Build history of the part. All positions in model axes, mm. A direction names the side the tool comes from. Round coordinates to 2 decimals unless told otherwise and drop trailing zeros. Write each loop counter-clockwise with the first axis right and the second up, starting at its lowest first coordinate (ties: lowest second). Pieces come first, ordered by that corner, then holes.
from build123d import *

# Parameters (mm, degrees)
F0_R     = 3
F1_DEPTH = 7.5
F0_R_2   = 2.35
F2_DEPTH = 7
F3_DEPTH = 0.5
F4_DEPTH = 7
F5_DEPTH = 0.5


with BuildPart() as f1:
    # F0 (on Top) → F1 (new body)
    with BuildSketch(Plane.XY):
        with BuildLine():
            ThreePointArc((-61.751105, -13.001984), (-60.682045, -15.582924), (-58.101105, -16.651984))
            Line((-58.101105, -16.651984), (5.748895, -16.651984))
            ThreePointArc((5.748895, -16.651984), (8.329835, -15.582924), (9.398895, -13.001984))
            ThreePointArc((9.398895, -13.001984), (8.329835, -10.421045), (5.748895, -9.351984))
            Line((5.748895, -9.351984), (-58.101105, -9.351984))
            ThreePointArc((-58.101105, -9.351984), (-60.682045, -10.421045), (-61.751105, -13.001984))
        make_face()
        with Locations((-58.101105, -13.001984)):
            Circle(F0_R, mode=Mode.SUBTRACT)
        with Locations((-50.101105, -13.001984)):
            Circle(F0_R, mode=Mode.SUBTRACT)
        with Locations((-42.101105, -13.001984)):
            Circle(F0_R, mode=Mode.SUBTRACT)
        with Locations((-34.101105, -13.001984)):
            Circle(F0_R, mode=Mode.SUBTRACT)
        with Locations((-26.101105, -13.001984)):
            Circle(F0_R, mode=Mode.SUBTRACT)
        with Locations((-18.101105, -13.001984)):
            Circle(F0_R, mode=Mode.SUBTRACT)
        with Locations((-10.101105, -13.001984)):
            Circle(F0_R, mode=Mode.SUBTRACT)
        with Locations((-2.101105, -13.001984)):
            Circle(F0_R, mode=Mode.SUBTRACT)
        with Locations((5.898895, -13.001984)):
            Circle(F0_R, mode=Mode.SUBTRACT)
    extrude(amount=F1_DEPTH)

    # F0 (on Top) → F2 (join)
    with BuildSketch(Plane.XY):
        with Locations((5.898895, -13.001984)):
            Circle(F0_R)
        with Locations((5.898895, -13.001984)):
            Circle(F0_R_2, mode=Mode.SUBTRACT)
    extrude(amount=F2_DEPTH)

    # F0 (on Top) → F3 (cut)
    with BuildSketch(Plane.XY):
        with Locations((5.898895, -13.001984)):
            Circle(F0_R)
        with Locations((5.898895, -13.001984)):
            Circle(F0_R_2, mode=Mode.SUBTRACT)
    extrude(amount=F3_DEPTH, mode=Mode.SUBTRACT)

    # F0 (on Top) → F4 (join)
    with BuildSketch(Plane.XY):
        with Locations((-58.101105, -13.001984)):
            Circle(F0_R)
        with Locations((-58.101105, -13.001984)):
            Circle(F0_R_2, mode=Mode.SUBTRACT)
        with Locations((-50.101105, -13.001984)):
            Circle(F0_R)
        with Locations((-50.101105, -13.001984)):
            Circle(F0_R_2, mode=Mode.SUBTRACT)
        with Locations((-42.101105, -13.001984)):
            Circle(F0_R)
        with Locations((-42.101105, -13.001984)):
            Circle(F0_R_2, mode=Mode.SUBTRACT)
        with Locations((-34.101105, -13.001984)):
            Circle(F0_R)
        with Locations((-34.101105, -13.001984)):
            Circle(F0_R_2, mode=Mode.SUBTRACT)
        with Locations((-26.101105, -13.001984)):
            Circle(F0_R)
        with Locations((-26.101105, -13.001984)):
            Circle(F0_R_2, mode=Mode.SUBTRACT)
        with Locations((-18.101105, -13.001984)):
            Circle(F0_R)
        with Locations((-18.101105, -13.001984)):
            Circle(F0_R_2, mode=Mode.SUBTRACT)
        with Locations((-10.101105, -13.001984)):
            Circle(F0_R)
        with Locations((-10.101105, -13.001984)):
            Circle(F0_R_2, mode=Mode.SUBTRACT)
        with Locations((-2.101105, -13.001984)):
            Circle(F0_R)
        with Locations((-2.101105, -13.001984)):
            Circle(F0_R_2, mode=Mode.SUBTRACT)
    extrude(amount=F4_DEPTH)

    # F0 (on Top) → F5 (cut)
    with BuildSketch(Plane.XY):
        with Locations((-58.101105, -13.001984)):
            Circle(F0_R)
        with Locations((-58.101105, -13.001984)):
            Circle(F0_R_2, mode=Mode.SUBTRACT)
        with Locations((-50.101105, -13.001984)):
            Circle(F0_R)
        with Locations((-50.101105, -13.001984)):
            Circle(F0_R_2, mode=Mode.SUBTRACT)
        with Locations((-42.101105, -13.001984)):
            Circle(F0_R)
        with Locations((-42.101105, -13.001984)):
            Circle(F0_R_2, mode=Mode.SUBTRACT)
        with Locations((-34.101105, -13.001984)):
            Circle(F0_R)
        with Locations((-34.101105, -13.001984)):
            Circle(F0_R_2, mode=Mode.SUBTRACT)
        with Locations((-26.101105, -13.001984)):
            Circle(F0_R_2)
        with Locations((-18.101105, -13.001984)):
            Circle(F0_R)
        with Locations((-18.101105, -13.001984)):
            Circle(F0_R_2, mode=Mode.SUBTRACT)
        with Locations((-10.101105, -13.001984)):
            Circle(F0_R)
        with Locations((-10.101105, -13.001984)):
            Circle(F0_R_2, mode=Mode.SUBTRACT)
        with Locations((-2.101105, -13.001984)):
            Circle(F0_R)
        with Locations((-2.101105, -13.001984)):
            Circle(F0_R_2, mode=Mode.SUBTRACT)
        with Locations((-26.101105, -13.001984)):
            Circle(F0_R)
        with Locations((-26.101105, -13.001984)):
            Circle(F0_R_2, mode=Mode.SUBTRACT)
    extrude(amount=F5_DEPTH, mode=Mode.SUBTRACT)


solid = f1.part
1) Slice it at A-A (x = -51). Write the cut outline in (y, z), plus the area to 3 significant figures.
Results:
outline: (-16.65, 0) - (-15.86, 0) - (-15.86, 0.5) - (-15.17, 0.5) - (-15.17, 7) - (-15.86, 7) - (-15.86, 7.5) - (-16.65, 7.5) - close; (-10.83, 0.5) - (-10.14, 0.5) - (-10.14, 0) - (-9.35, 0) - (-9.35, 7.5) - (-10.14, 7.5) - (-10.14, 7) - (-10.83, 7) - close
area: 20.8 mm2
2) Slice it at C-C (x = -32.5). Write the cut outline in (y, z).
Results:
outline: (-16.65, 0) - (-15.54, 0) - (-15.54, 0.5) - (-14.72, 0.5) - (-14.72, 7) - (-15.54, 7) - (-15.54, 7.5) - (-16.65, 7.5) - close; (-11.28, 0.5) - (-10.46, 0.5) - (-10.46, 0) - (-9.35, 0) - (-9.35, 7.5) - (-10.46, 7.5) - (-10.46, 7) - (-11.28, 7) - close
3) Wall check: L1, parallel to Z at x = -34, y = -10.25; L2, parallel to Y at x = -57, z = 6.5; L3, parallel to Y at x = -36, z = 6. Give the ranges that are in metal, low to high.
Results:
L1: z = 0.5 to 7
L2: y = -16.65 to -15.08, -10.93 to -9.35
L3: y = -16.65 to -14.39, -11.62 to -9.35
4) Mould opens along Y. For faces 4 (the flat face through (4, -15, 7)), 5 (the flat face through (-23.7, -10.6, 0)) say: released by +Y, released by -Y, zero draft, split by the parting line, or undercut.
Results:
face 4: undercut
face 5: zero draft
5) Pin check, flat tips, straight feed: pin 1 Ø1.5 at (x, y) = (-24.5, -11.5) entering from +Z; pin 2 Ø3 at (x, y) = (-26.5, -13.5) entering from +Z; pin 3 Ø1.5 at (y, z) = (-12, 6.5) entering from +X. Stop position of each tip, or through.
Results:
pin 1: stops at z = 7
pin 2: passes through
pin 3: stops at x = 9.39
6) Which spindle directions (+Z, -Z, +X, -X, +Y, -Y) get a long thin tool onto all of the face, cutting with end or side? Do faces 1 (the cylindrical face through (-60.45, -12.9, 3.7)), 2 (the flat face through (-20, -15, 0.5)), 3 (the flat face through (-36, -15, 7)). Say none if no direction does.
Results:
face 1: +Z, -Z
face 2: -Z
face 3: +Z
7) Slice it at B-B (z = 2.5). Count the separate pieces of the cut face and the enclosed holes in it, plus the area to 3 significant figures.
Results:
separate pieces: 1
enclosed holes: 9
area: 352 mm2
